from build123d import *

# Parameters (mm, degrees)
SKETCH2_R               = 62.5
BOSS_EXTRUDE1_DEPTH     = 50
CUT_EXTRUDE1_DEPTH      = 63.5
CUT_EXTRUDE1_DEPTH_BACK = 63.5
SKETCH4_R               = 30
BOSS_EXTRUDE2_DEPTH     = 50
SKETCH5_R               = 50
CUT_EXTRUDE2_DEPTH      = 33.808019269
CUT_EXTRUDE2_DEPTH_BACK = 10
BOSS_EXTRUDE3_DEPTH     = 40


with BuildPart() as part:
    # Sketch2 → Boss-Extrude1 (new body)
    with BuildSketch(Plane(origin=(0, 0, 0), x_dir=(1, 0, 0), z_dir=(0, 1, 0))):
        Circle(SKETCH2_R)
    extrude(amount=BOSS_EXTRUDE1_DEPTH)

    # Sketch3 → Cut-Extrude1 (cut, two sides)
    with BuildSketch(Plane(origin=(0, 0, 0), x_dir=(0, 0, -1), z_dir=(1, 0, 0))) as cut_extrude1_sk:
        Polygon((-62.5, 0), (62.5, 34), (62.5, 0), align=None)
    extrude(amount=CUT_EXTRUDE1_DEPTH, mode=Mode.SUBTRACT)
    extrude(cut_extrude1_sk.sketch, amount=-CUT_EXTRUDE1_DEPTH_BACK, mode=Mode.SUBTRACT)

    # Sketch4 → Boss-Extrude2 (add)
    with BuildSketch(Plane(origin=(0, 50, 0), x_dir=(1, 0, 0), z_dir=(0, 1, 0))):
        Circle(SKETCH4_R)
    extrude(amount=BOSS_EXTRUDE2_DEPTH)

    # Sketch5 → Cut-Extrude2 (cut, two sides)
    with BuildSketch(Plane(origin=(0, 15.828913652, 4.305464513), x_dir=(1, 0, 0), z_dir=(0, -0.964941743, -0.262464154))) as cut_extrude2_sk:
        with Locations((0, -4.461890621)):
            Circle(SKETCH5_R)
    extrude(amount=CUT_EXTRUDE2_DEPTH, mode=Mode.SUBTRACT)
    extrude(cut_extrude2_sk.sketch, amount=-CUT_EXTRUDE2_DEPTH_BACK, mode=Mode.SUBTRACT)

    # Sketch7 → Revolve1 (revolve)
    with BuildSketch(Plane(origin=(0, 0, 0), x_dir=(0, 0, -1), z_dir=(1, 0, 0))):
        Polygon((-50.871728702, 13.526209724), (-1.273723101, 14.062717334), (0.656160385, 14.587645642), (-2.624641542, 26.649417432), align=None)
    revolve(axis=Axis((0, 14.587645642, -0.656160385), (0, 0.964941743, 0.262464154)))

    # Sketch8 → Boss-Extrude3 (add)
    with BuildSketch(Plane(origin=(0, 50, 0), x_dir=(1, 0, 0), z_dir=(0, 1, 0))):
        with BuildLine():
            Line((25.321153679, 57.140958833), (67.747560551, 99.567365704))
            Line((67.747560551, 99.567365704), (99.567365704, 67.747560551))
            Line((99.567365704, 67.747560551), (57.140958833, 25.321153679))
            ThreePointArc((57.140958833, 25.321153679), (44.194173824, 44.194173824), (25.321153679, 57.140958833))
        make_face()
    extrude(amount=-BOSS_EXTRUDE3_DEPTH)


solid = part.part
Read the model definition and answer for the solid it produces. Units are mm, in the model's axes. A direction names the side the tool comes from. Give positions to 0.01 mm unless a question says otherwise; leave off trailing zeros. Loops run counter-clockwise (first coordinate to the right, second up) from the corner with the lowest first, then second, coordinate; pieces in that order, holes last. Notation, with made-up numbers: (-21.75, -5) - (-16.75, -5) arc R22 ccw to (-16.75, 17) - close; hole circle Ø8 at (8, -2). An arc over 180 degrees is marked (long way). Answer as CSV lines item,"result". Start each with the question number.
1) Which of the six approach directions +Z, -Z, +X, -X, +Y, -Y give full straight-line access (tool end or side, diameter ignored) to faces 5 (the face through (0, 14.6, -0.7)), 6 (the face through (38, 50, -20)), 7 (the face through (44.42, 18.92, -43.97))?
2) Find section C-C (x = 80). Write down the section's boundary in (y, z).
3) Straight lines are drawn through the part: L1, parallel to Z at x = 34, y = 32.5; L2, parallel to Y at x = -28, z = 55; L3, parallel to X at y = 29, z = -64.5. For each, find the intervals that lie inside material, in ascending order. Write a range as from..to.
4) Determine the mould class of faces 1 (the face through (47.69, 17.82, 15.79)), 2 (the face through (63, 10, -63)), 3 (the face through (-4.23, 15.42, -1.4)), 4 (the face through (-29.97, 74.65, -1.32)) for opening direction X: released by +X, released by -X, zero draft, split by the parting line, or undercut.
5) Each of these flat-tipped pins is pushed along its axis until it touches: pin 1 Ø1.5 at (x, z) = (12.5, -43) entering from -Y; pin 2 Ø5 at (x, y) = (-40, 42.5) entering from -Z; pin 3 Ø8 at (x, y) = (-3, 70.5) entering from -Z. Where does it stop, or does it pass through?
6) Find section B-B (z = -81). Write down the section's boundary in (x, y), then the cut area to 3 significant figures.
7) Find section A-A (y = 89.5). Write down the section's boundary in (x, z), then the cut area to 3 significant figures.
Findings below:
1,face 5,"-Z, +X, -X, -Y"
1,face 6,"+Y"
1,face 7,"-X, -Y"
2,outline,"(10, -87.31) - (50, -87.31) - (50, -48.18) - (10, -48.18) - close"
3,L1,"-65.82..-33.78, -24.8..52.44"
3,L2,"2.04..50"
3,L3,"32.68..96.32"
4,face 1,"undercut"
4,face 2,"zero draft"
4,face 3,"undercut"
4,face 4,"split by the parting line"
5,pin 1,"y = 38.32"
5,pin 2,"z = -50"
5,pin 3,"z = -30"
6,outline,"(49.18, 10) - (86.31, 10) - (86.31, 50) - (49.18, 50) - close"
6,area,"1,490 mm^2"
7,outline,"circle Ø60 at (0, 0)"
7,area,"2,830 mm^2"
